Check sheet for the drawn part. Datum: minimum x, y, z corner. Units: mm. Round coordinates to 2 decimals unless told otherwise and drop trailing zeros. Write each loop counter-clockwise with the first axis right and the second up, starting at its lowest first coordinate (ties: lowest second). Pieces come first, ordered by that corner, then holes. Notation, with made-up numbers: M 3,37.5 L 35,37.5 A19 cw 35,68.5 Z; hole C -17,71 d3. An arc over 180 degrees is marked long. One line per item, written item: value. Start each with the question number.
Item 1: Gauge pin test, flat ends, axial feed: pin 1 (2 mm diameter, centred on y = 113.5, z = 4.5, fed in from +X) (1 decimal); pin 2 (1.9 mm diameter, centred on y = 165.5, z = 4, fed in from +X); pin 3 (3 mm diameter, centred on y = 23.5, z = 4.5, fed in from -X). Record the tip position at first contact, or that the pin passes through.
Item 2: Section check C-C, the plane x = 12.5. Record the cut outline in (y, z), then the cut area to 3 significant figures.
Item 3: Thickness scan on probe 1 along X at (y, z) = (20.5, 3.5) (1 decimal); probe 2 along X at (y, z) = (35, 4.5); probe 3 along X at (y, z) = (70, 3.75) (1 decimal). Record the ranges inside material, lowest first. Write a range as from..to.
Item 4: Section check A-A, the plane y = 20.32. Record the cut outline in (x, z).
Item 5: Section check D-D, the plane y = 75.5. Record the cut outline in (x, z).
Item 6: Section check B-B, the plane z = 3. Record the cut outline in (x, y) (1 decimal), then the cut area to 3 significant figures.
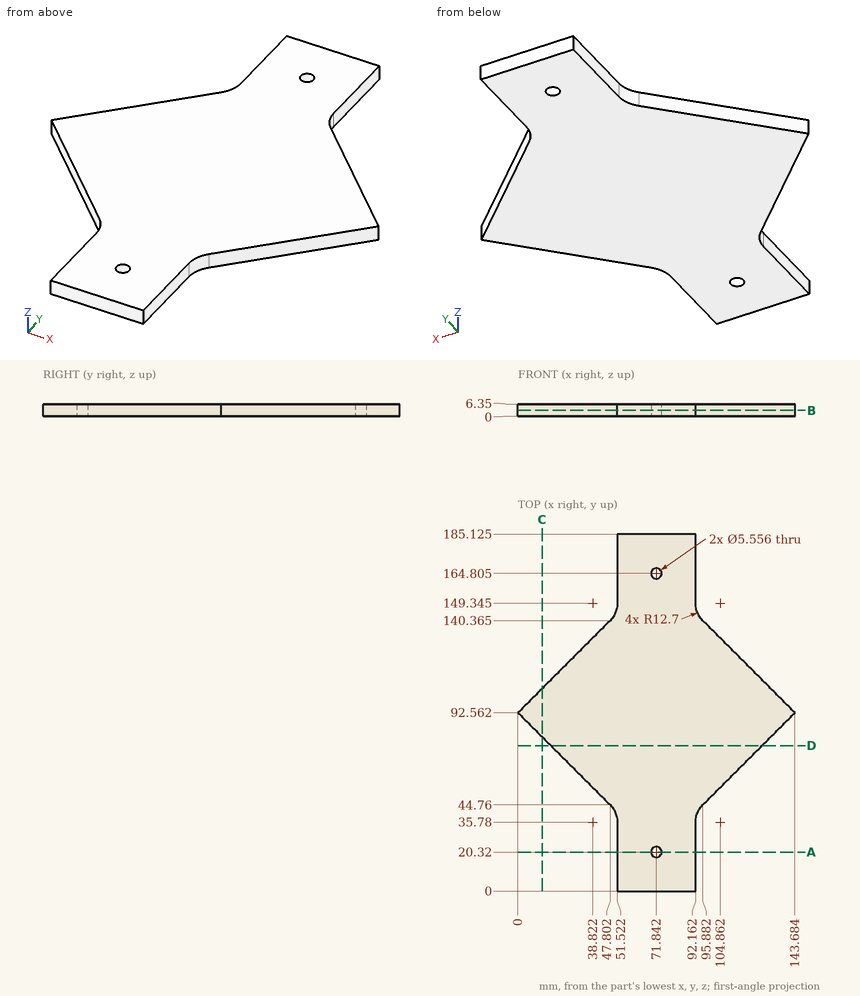
Response values:
1. pin 1: stops at x = 123.7
1. pin 2: stops at x = 92.16
1. pin 3: stops at x = 51.52
2. outline: M 80.06,0 L 105.06,0 L 105.06,6.35 L 80.06,6.35 Z
2. area: 159 mm2
3. probe 1: x = 51.5..69.1, 74.6..92.2
3. probe 2: x = 51.52..92.16
3. probe 3: x = 22.6..121.1
4. outline: M 51.52,0 L 69.06,0 L 69.06,6.35 L 51.52,6.35 Z; M 74.62,0 L 92.16,0 L 92.16,6.35 L 74.62,6.35 Z
5. outline: M 17.06,0 L 126.62,0 L 126.62,6.35 L 17.06,6.35 Z
6. outline: M 0,92.6 L 47.8,44.8 A12.7 cw 51.5,35.8 L 51.5,0 L 92.2,0 L 92.2,35.8 A12.7 cw 95.9,44.8 L 143.7,92.6 L 95.9,140.4 A12.7 cw 92.2,149.3 L 92.2,185.1 L 51.5,185.1 L 51.5,149.3 A12.7 cw 47.8,140.4 Z; hole C 71.8,20.3 d5.6; hole C 71.8,164.8 d5.6
6. area: 12,800 mm2
